Source: CAD feature listing. Evaluate the final solid. Frame: model axes, mm. Face numbers are marked on the shaded views. A direction names the side the tool comes from. Give positions to 0.01 mm unless a question says otherwise; leave off trailing zeros. Loops run counter-clockwise (first coordinate to the right, second up) from the corner with the lowest first, then second, coordinate; pieces in that order, holes last.
from build123d import *

# Parameters (mm, degrees)
SKICA1_W                 = 50
SKICA1_H                 = 25
P_IDAT_VYSUNUT_M1_DEPTH  = 10
P_IDAT_VYSUNUT_M2_DEPTH  = 10
SKICA3_R                 = 2.1
ODEBRAT_VYSUNUT_M1_DEPTH = 10
ODEBRAT_VYSUNUT_M2_DEPTH = 10
SKICA5_R                 = 2.1
ODEBRAT_VYSUNUT_M3_DEPTH = 10
SKICA6_W                 = 15
SKICA6_H                 = 10
P_IDAT_VYSUNUT_M3_DEPTH  = 5
ODEBRAT_VYSUNUT_M5_DEPTH = 3.5
ODEBRAT_VYSUNUT_M6_DEPTH = 4
ZKOSEN_1_SIZE            = 10
ODEBRAT_VYSUNUT_M7_DEPTH = 5
ZKOSEN_3_SIZE            = 1
ZKOSEN_4_SIZE            = 0.5
ZKOSEN_5_SIZE            = 1
ZKOSEN_7_SIZE            = 1


with BuildPart() as part:
    # Skica1 → Přidat vysunutím1 (new body)
    with BuildSketch(Plane.XY):
        with Locations((25, 12.5)):
            Rectangle(SKICA1_W, SKICA1_H)
    extrude(amount=P_IDAT_VYSUNUT_M1_DEPTH)

    # Skica2 → Přidat vysunutím2 (add)
    with BuildSketch(Plane.XY.offset(10)):
        Polygon((0, 0), (35, 0), (50, 15.532954707), (50, 25), (44, 25), (44, 17.957112062), (32.453151103, 6), (0, 6), align=None)
    extrude(amount=P_IDAT_VYSUNUT_M2_DEPTH)

    # Skica3 → Odebrat vysunutím1 (cut)
    with BuildSketch(Plane.XY.offset(10)):
        with Locations((6, 19)):
            Circle(SKICA3_R)
    extrude(amount=-ODEBRAT_VYSUNUT_M1_DEPTH, mode=Mode.SUBTRACT)

    # Skica4 → Odebrat vysunutím2 (cut)
    with BuildSketch(Plane.XY.offset(10)):
        Polygon((50, 15.532954707), (35, 0), (50, 0), align=None)
    extrude(amount=-ODEBRAT_VYSUNUT_M2_DEPTH, mode=Mode.SUBTRACT)

    # Skica5 → Odebrat vysunutím3 (cut)
    with BuildSketch(Plane(origin=(18.110741192, -17.489339473, 0), x_dir=(0, 0, -1), z_dir=(0.7193398003386524, -0.6946583704589961, 0))):
        with Locations(Location((-15, 32.313042966, 0), (0, 0, 90))):
            Circle(SKICA5_R)
    extrude(amount=-ODEBRAT_VYSUNUT_M3_DEPTH, mode=Mode.SUBTRACT)

    # Skica6 → Přidat vysunutím3 (add)
    with BuildSketch(Plane(origin=(0, 25, 0), x_dir=(1, 0, 0), z_dir=(0, 1, 0))):
        with Locations((-7.5, -5)):
            Rectangle(SKICA6_W, SKICA6_H)
        with Locations((57.5, -5)):
            Rectangle(SKICA6_W, SKICA6_H)
    extrude(amount=-P_IDAT_VYSUNUT_M3_DEPTH)

    # Skica9 → Odebrat vysunutím5 (cut)
    with BuildSketch(Plane(origin=(18.110741192, -17.489339473, 0), x_dir=(0, 0, -1), z_dir=(0.7193398003386524, -0.6946583704589961, 0))):
        Polygon((-19.156921938, 32.313042966), (-17.078460969, 28.713042966), (-12.921539031, 28.713042966), (-10.843078062, 32.313042966), (-12.921539031, 35.913042966), (-17.078460969, 35.913042966), align=None)
    extrude(amount=-ODEBRAT_VYSUNUT_M5_DEPTH, mode=Mode.SUBTRACT)

    # Skica10 → Odebrat vysunutím6 (cut)
    with BuildSketch(Plane(origin=(0, 0, 0), x_dir=(-1, 0, 0), z_dir=(0, 0, -1))):
        Polygon((-6, 23.156921938), (-9.6, 21.078460969), (-9.6, 16.921539031), (-6, 14.843078062), (-2.4, 16.921539031), (-2.4, 21.078460969), align=None)
    extrude(amount=-ODEBRAT_VYSUNUT_M6_DEPTH, mode=Mode.SUBTRACT)

    # Zkosení1
    zkosen_1_edges = [part.edges().sort_by_distance(p)[0] for p in [
        (0, 3, 20),
    ]]
    chamfer(zkosen_1_edges, length=ZKOSEN_1_SIZE)

    # Skica11 → Odebrat vysunutím7 (cut)
    with BuildSketch(Plane.XZ.offset(-20)):
        with BuildLine():
            Line((-10, 7.1), (-5, 7.1))
            ThreePointArc((-5, 7.1), (-2.9, 5), (-5, 2.9))
            Line((-5, 2.9), (-10, 2.9))
            ThreePointArc((-10, 2.9), (-12.1, 5), (-10, 7.1))
        make_face()
        with BuildLine():
            Line((55, 7.1), (60, 7.1))
            ThreePointArc((60, 7.1), (62.1, 5), (60, 2.9))
            Line((60, 2.9), (55, 2.9))
            ThreePointArc((55, 2.9), (52.9, 5), (55, 7.1))
        make_face()
    extrude(amount=-ODEBRAT_VYSUNUT_M7_DEPTH, mode=Mode.SUBTRACT)

    # Zkosení3
    zkosen_3_edges = [part.edges().sort_by_distance(p)[0] for p in [
        (44, 21.478556031, 10),
        (38.226575551, 11.978556031, 10),
        (16.226575551, 6, 10),
    ]]
    chamfer(zkosen_3_edges, length=ZKOSEN_3_SIZE)

    # Zkosení4
    zkosen_4_edges = [part.edges().sort_by_distance(p)[0] for p in [
        (22.5, 0, 20),
        (5, 0, 15),
        (5.5, 6, 15.5),
        (42.5, 7.766477353, 20),
        (50, 20.266477353, 20),
        (47, 25, 20),
        (44, 21.478556031, 20),
        (38.226575551, 11.978556031, 20),
        (21.226575551, 6, 20),
    ]]
    chamfer(zkosen_4_edges, length=ZKOSEN_4_SIZE)

    # Zkosení5
    zkosen_5_edges = [part.edges().sort_by_distance(p)[0] for p in [
        (0, 20, 5),
        (50, 20, 5),
    ]]
    chamfer(zkosen_5_edges, length=ZKOSEN_5_SIZE)

    # Zkosení7
    zkosen_7_edges = [part.edges().sort_by_distance(p)[0] for p in [
        (-15, 22.5, 10),
        (-15, 22.5, 0),
        (65, 22.5, 0),
        (65, 22.5, 10),
    ]]
    chamfer(zkosen_7_edges, length=ZKOSEN_7_SIZE)


solid = part.part
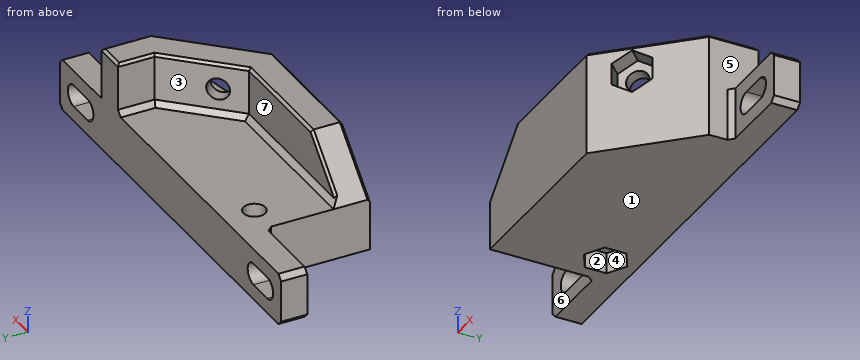
1) Cut plane B-B (x = -8). Return loops of the section in (y, z).
Checks:
outline: (20, 0) - (25, 0) - (25, 2.9) - (20, 2.9) - close; (20, 7.1) - (25, 7.1) - (25, 10) - (20, 10) - close
2) Ray query, probe 1 along Y at (x, z) = (6, 5.85); probe 2 along Z at (x, y) = (15.5, 15); probe 3 along Z at (x, y) = (6.5, 15.5). Return the intervals inside material, ascending.
Checks:
probe 1: y = 0 to 16.9, 21.1 to 25
probe 2: z = 0 to 10
probe 3: z = 4 to 10
3) Reachability of the marked faces 5, 6 and 7 from +Z, -Z, +X, -X, +Y, -Y: full face, straight path, thin tool, end or side. Return the list, or none.
Checks:
face 5: +Z, +X, -Y
face 6: +Z, -Z, -X, -Y
face 7: +Z, -X, +Y
4) Cut plane A-A (z = 5). Return loops of the section in (x, y), and give its area (3 significant figures).
Checks:
outline: (-15, 20) - (-12.1, 20) - (-12.1, 25) - (-15, 25) - close; (-2.9, 20) - (-1, 20) - (0, 19) - (0, 0) - (35, 0) - (50, 15.53) - (50, 19) - (51, 20) - (52.9, 20) - (52.9, 25) - (-2.9, 25) - close; (62.1, 20) - (65, 20) - (65, 25) - (62.1, 25) - close; hole circle Ø4.2 at (6, 19)
area: 1,180 mm2
5) Pull-direction query (X, two-part tool) for the marked faces 1, 2, 3 and 4; classes: released by +X, released by -X, zero draft, split by the parting line, or undercut.
Checks:
face 1: zero draft
face 2: undercut
face 3: released by -X
face 4: undercut
6) Contact query for flat-ended pins moving along their axis: P1, Ø5.5, axis at x = -6.5, y = 23, coming from the +Z side; P2, Ø2, axis at x = 25, z = 13.5, coming from the +Y side; P3, Ø6, axis at y = 14.5, z = 10, coming from the -X side; P4, Ø3.5, axis at x = 6, y = 19, coming from the +Z side. Output: stop coordinate, or through.
Checks:
P1: stops at z = 10
P2: stops at y = 6
P3: stops at x = 0
P4: passes through
